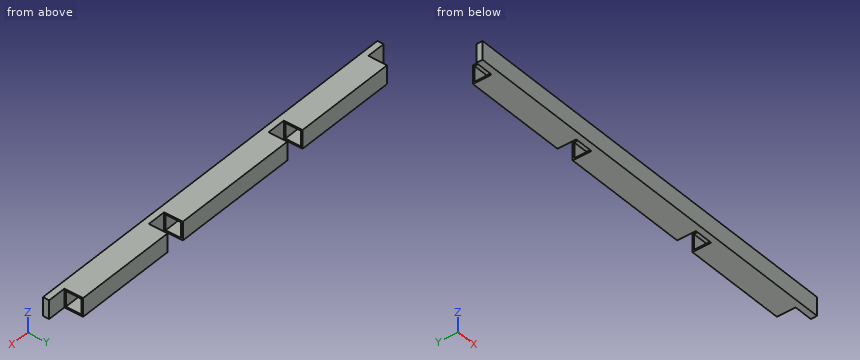
```python
from build123d import *

# Parameters (mm, degrees)
SKETCH1_W           = 838.1
SKETCH1_H           = 12.7
BOSS_EXTRUDE1_DEPTH = 38.1
SKETCH2_W           = 211.9
SKETCH2_H           = 38.1
SKETCH2_W_2         = 261.9
BOSS_EXTRUDE2_DEPTH = 38.1
SKETCH6_W           = 31.75
SKETCH6_H           = 31.75
CUT_EXTRUDE2_DEPTH  = 801


with BuildPart() as part:
    # Sketch1 → Boss-Extrude1 (new body)
    with BuildSketch(Plane.XY):
        with Locations((419.05, 6.35)):
            Rectangle(SKETCH1_W, SKETCH1_H)
    extrude(amount=-BOSS_EXTRUDE1_DEPTH)

    # Sketch2 → Boss-Extrude2 (add)
    with BuildSketch(Plane(origin=(0, 12.7, 0), x_dir=(1, 0, 0), z_dir=(0, 1, 0))):
        with Locations((144.05, 19.05)):
            Rectangle(SKETCH2_W, SKETCH2_H)
        with Locations((419.05, 19.05)):
            Rectangle(SKETCH2_W_2, SKETCH2_H)
        with Locations((694.05, 19.05)):
            Rectangle(SKETCH2_W, SKETCH2_H)
    extrude(amount=BOSS_EXTRUDE2_DEPTH)

    # Sketch6 → Cut-Extrude2 (cut, through all)
    with BuildSketch(Plane.ZY.offset(-38.1)):
        with Locations((-19.05, 31.75)):
            Rectangle(SKETCH6_W, SKETCH6_H)
    extrude(amount=-CUT_EXTRUDE2_DEPTH, mode=Mode.SUBTRACT)


solid = part.part
```
Check sheet for the modelled part. Datum: model origin and axes. Units: mm. Give positions to 0.01 mm unless a question says otherwise; leave off trailing zeros. Write each loop counter-clockwise with the first axis right and the second up, starting at its lowest first coordinate (ties: lowest second). Pieces come first, ordered by that corner, then holes.
Item 1: Gauge pin test, flat ends, axial feed: pin 1 (19 mm diameter, centred on y = 24, z = -17, fed in from -X); pin 2 (11.5 mm diameter, centred on y = 22.5, z = -28, fed in from +X). Record the tip position at first contact, or that the pin passes through.
Item 2: Cross-section at B-B (z = -12). Enter the section's corners in (x, y) (3 decimals), and give its area (3 significant figures).
Item 3: Cross-section at A-A (y = 33.5). Enter the section's corners in (x, z) (3 decimals), and give its area (3 significant figures).
Item 4: Scan lines: L1, parallel to X at y = 42.5, z = -37; L2, parallel to Y at x = 360.5, z = -7.5 (3 decimals); L3, parallel to Z at x = 370, y = 39 (3 decimals). Record each from-to range of solid material in increasing order.
Item 5: Cross-section at C-C (x = 103.5). Enter the section's corners in (y, z) (3 decimals), and give its area (3 significant figures).
Report:
1. pin 1: stops at x = 38.1
1. pin 2: passes through
2. outline: (0, 0) - (838.1, 0) - (838.1, 12.7) - (800, 12.7) - (800, 15.875) - (588.1, 15.875) - (588.1, 12.7) - (550, 12.7) - (550, 15.875) - (288.1, 15.875) - (288.1, 12.7) - (250, 12.7) - (250, 15.875) - (38.1, 15.875) - (38.1, 12.7) - (0, 12.7) - close; (38.1, 47.625) - (250, 47.625) - (250, 50.8) - (38.1, 50.8) - close; (288.1, 47.625) - (550, 47.625) - (550, 50.8) - (288.1, 50.8) - close; (588.1, 47.625) - (800, 47.625) - (800, 50.8) - (588.1, 50.8) - close
2. area: 15,000 mm2
3. outline: (38.1, -38.1) - (250, -38.1) - (250, -34.925) - (38.1, -34.925) - close; (38.1, -3.175) - (250, -3.175) - (250, 0) - (38.1, 0) - close; (288.1, -38.1) - (550, -38.1) - (550, -34.925) - (288.1, -34.925) - close; (288.1, -3.175) - (550, -3.175) - (550, 0) - (288.1, 0) - close; (588.1, -38.1) - (800, -38.1) - (800, -34.925) - (588.1, -34.925) - close; (588.1, -3.175) - (800, -3.175) - (800, 0) - (588.1, 0) - close
3. area: 4,350 mm2
4. L1: x = 38.1 to 250, 288.1 to 550, 588.1 to 800
4. L2: y = 0 to 15.875, 47.625 to 50.8
4. L3: z = -38.1 to -34.925, -3.175 to 0
5. outline: (0, -38.1) - (50.8, -38.1) - (50.8, 0) - (0, 0) - close; hole (15.875, -34.925) - (47.625, -34.925) - (47.625, -3.175) - (15.875, -3.175) - close
5. area: 927 mm2
